Source: CAD feature listing. Evaluate the final solid. Frame: model axes, mm. A direction names the side the tool comes from. Give positions to 0.01 mm unless a question says otherwise; leave off trailing zeros. Loops run counter-clockwise (first coordinate to the right, second up) from the corner with the lowest first, then second, coordinate; pieces in that order, holes last. Notation, with made-up numbers: M 89,72.5 L 105,72.5 A32 cw 105,100.5 Z; hole C 38,55.5 d8. An arc over 180 degrees is marked long. Answer in a Markdown table with one row per item.
```python
from build123d import *

# Parameters (mm, degrees)
ESBO_O1_R                  = 10
RESSALTO_EXTRUS_O1_DEPTH   = 17
ESBO_O4_R                  = 7.5
CORTE_EXTRUS_O3_DEPTH      = 10
CORTE_EXTRUS_O1_START      = -5
CORTE_EXTRUS_O1_DEPTH      = 5
CORTE_EXTRUS_O4_REACH      = 26.779
CORTE_EXTRUS_O4_END_RADIUS = 10
ESBO_O5_R                  = 1.5


with BuildPart() as part:
    # Esboço1 → Ressalto-extrusão1 (new body)
    with BuildSketch(Plane.XY):
        Circle(ESBO_O1_R)
    extrude(amount=RESSALTO_EXTRUS_O1_DEPTH)

    # Esboço4 → Corte-extrusão3 (cut)
    with BuildSketch(Plane(origin=(0, 0, 0), x_dir=(-1, 0, 0), z_dir=(0, 0, -1))):
        Circle(ESBO_O4_R)
    extrude(amount=-CORTE_EXTRUS_O3_DEPTH, mode=Mode.SUBTRACT)

    # Esboço2 → Corte-extrusão1 (cut)
    with BuildSketch(Plane.XY.offset(17).offset(CORTE_EXTRUS_O1_START)):
        with BuildLine():
            Line((-5, 8.660254038), (-5, -8.660254038))
            ThreePointArc((-5, -8.660254038), (-10, 0), (-5, 8.660254038))
        make_face()
        with BuildLine():
            Line((5, 8.660254038), (5, -8.660254038))
            ThreePointArc((5, -8.660254038), (10, 0), (5, 8.660254038))
        make_face()
    extrude(amount=CORTE_EXTRUS_O1_DEPTH, mode=Mode.SUBTRACT)

    # Corte-extrusão4: up to this cylinder (the profile starts inside it)
    corte_extrus_o4_end = Plane(origin=(0, 0, 5), z_dir=(0, 0, -1)) * Cylinder(CORTE_EXTRUS_O4_END_RADIUS, 74.558, mode=Mode.PRIVATE)
    # Esboço5 → Corte-extrusão4 (cut, up to the surface)
    with BuildSketch(Plane(origin=(5, 0, 0), x_dir=(0, 0, -1), z_dir=(1, 0, 0)), mode=Mode.PRIVATE) as corte_extrus_o4_sk1:
        with Locations(Location((-5, 0, 0), (0, 0, 270))):
            Circle(ESBO_O5_R)
    corte_extrus_o4_tool1 = extrude(corte_extrus_o4_sk1.sketch, amount=CORTE_EXTRUS_O4_REACH, mode=Mode.PRIVATE) & corte_extrus_o4_end
    add(corte_extrus_o4_tool1.solids().sort_by_distance((5, 0, 5))[0], mode=Mode.SUBTRACT)


solid = part.part
```
1) Material intervals for L1, parallel to Y at x = 0, z = 4.25; L2, parallel to X at y = -6, z = 12.25; L3, parallel to Z at x = -0.5, y = -2, sorted ascending.
Reply:
| item | result |
|---|---|
| L1 | y = -10 to -7.5, 7.5 to 10 |
| L2 | x = -5 to 5 |
| L3 | z = 10 to 17 |
2) Section B-B, the plane x = 0. Return loops of the section in (y, z), then the cut area to 3 significant figures.
Reply:
| item | result |
|---|---|
| outline | M -10,0 L -7.5,0 L -7.5,10 L 7.5,10 L 7.5,0 L 10,0 L 10,17 L -10,17 Z |
| area | 190 mm² |
3) Pull-direction query (X, two-part tool) for faces 6 (the cylindrical face through (4.614, -8.872, 6.492)), 7 (the flat face through (5, 0, 14)), 8 (the flat face through (0, 0, 10)), 9 (the cylindrical face through (8.66, -1.43, 4.55)); classes: released by +X, released by -X, zero draft, split by the parting line, or undercut.
Reply:
| item | result |
|---|---|
| face 6 | split by the parting line |
| face 7 | released by +X |
| face 8 | undercut |
| face 9 | zero draft |
4) Pin query (flat end, axial travel): pin 1 Ø4 at (x, y) = (1, 1) entering from -Z; pin 2 Ø5.5 at (y, z) = (-0.5, 15) entering from +X; pin 3 Ø2.5 at (y, z) = (0, 5) entering from +X. Return the tip coordinate at first contact, or that it passes through.
Reply:
| item | result |
|---|---|
| pin 1 | stops at z = 10 |
| pin 2 | stops at x = 5 |
| pin 3 | stops at x = -7.4 |
5) Section C-C, the plane y = 8. Return loops of the section in (x, z), then the cut area to 3 significant figures.
Reply:
| item | result |
|---|---|
| outline | M -6,0 L 6,0 L 6,12 L 5,12 L 5,17 L -5,17 L -5,12 L -6,12 Z |
| area | 194 mm² |
6) Set-up query: faces 1 (the flat face through (-7, 0, 12)), 2 (the flat face through (7, 0, 12)), 3 (the cylindrical face through (-6.93, -2.87, 4.93)), 4 (the flat face through (4, 7, 0)), 5 (the flat face through (0, 0, 17)). Return all of +Z, -Z, +X, -X, +Y, -Y with unobstructed straight access to the full face (end or side cutting, diameter ignored); none if empty.
Reply:
| item | result |
|---|---|
| face 1 | +Z, -X, +Y, -Y |
| face 2 | +Z, +X, +Y, -Y |
| face 3 | -Z |
| face 4 | -Z, +X, -X, +Y, -Y |
| face 5 | +Z, +X, -X, +Y, -Y |
7) Section D-D, the plane z = 2.5. Return loops of the section in (x, y), then the cut area to 3 significant figures.
Reply:
| item | result |
|---|---|
| outline | C 0,0 d20; hole C 0,0 d15 |
| area | 137 mm² |
8) Section A-A, the plane y = 0. Return loops of the section in (x, z), then the cut area to 4 significant figures.
Reply:
| item | result |
|---|---|
| outline | M -10,0 L -7.5,0 L -7.5,10 L 7.5,10 L 7.5,6.5 L 10,6.5 L 10,12 L 5,12 L 5,17 L -5,17 L -5,12 L -10,12 Z; M 7.5,0 L 10,0 L 10,3.5 L 7.5,3.5 Z |
| area | 132.5 mm² |
